Verification items for the finished model (mm, model axes). Face numbers are marked on the shaded views. A direction names the side the tool comes from. Give positions to 0.01 mm unless a question says otherwise; leave off trailing zeros. Write each loop counter-clockwise with the first axis right and the second up, starting at its lowest first coordinate (ties: lowest second). Pieces come first, ordered by that corner, then holes.
from build123d import *

# Parameters (mm, degrees)
BOSS_EXTRUDE1_DEPTH                  = 33.3375
SKETCH3_R                            = 2.0193
CUT_EXTRUDE1_DEPTH                   = 68.328625042
CUT_EXTRUDE3_START                   = -7.9375
SKETCH8_R                            = 6.875
SKETCH8_R_2                          = 6.35
CUT_EXTRUDE3_DEPTH                   = 7.9375
F_10_32_TAPPED_HOLE1_D               = 4.0386
F_10_32_TAPPED_HOLE1_DEPTH           = 12.02944
F_10_32_TAPPED_HOLE1_TIP             = 1.213317848
F_10_32_TAPPED_HOLE1_ON_FACE_2_D     = 4.0386
F_10_32_TAPPED_HOLE1_ON_FACE_2_DEPTH = 12.02944
F_10_32_TAPPED_HOLE1_ON_FACE_2_TIP   = 1.213317848


with BuildPart() as part:
    # Sketch1 → Boss-Extrude1 (new, symmetric)
    with BuildSketch(Plane.XY):
        with BuildLine():
            Line((-0.893039494, 6.816751826), (-5.456960506, 4.181770802))
            ThreePointArc((-5.456960506, 4.181770802), (-5.953924651, 3.4375), (-6.35, 2.634981025))
            Line((-6.35, 2.634981025), (-6.35, -2.634981025))
            ThreePointArc((-6.35, -2.634981025), (-5.953924651, -3.4375), (-5.456960506, -4.181770802))
            Line((-5.456960506, -4.181770802), (-0.893039494, -6.816751826))
            ThreePointArc((-0.893039494, -6.816751826), (0, -6.875), (0.893039494, -6.816751826))
            Line((0.893039494, -6.816751826), (5.456960506, -4.181770802))
            ThreePointArc((5.456960506, -4.181770802), (5.953924651, -3.4375), (6.35, -2.634981025))
            Line((6.35, -2.634981025), (6.35, 2.634981025))
            ThreePointArc((6.35, 2.634981025), (5.953924651, 3.4375), (5.456960506, 4.181770802))
            Line((5.456960506, 4.181770802), (0.893039494, 6.816751826))
            ThreePointArc((0.893039494, 6.816751826), (0, 6.875), (-0.893039494, 6.816751826))
        make_face()
    extrude(amount=BOSS_EXTRUDE1_DEPTH, both=True)

    # Sketch3 → Cut-Extrude1 (cut, through all)
    with BuildSketch(Plane.XY.offset(33.3375)):
        Circle(SKETCH3_R)
    extrude(amount=-CUT_EXTRUDE1_DEPTH, mode=Mode.SUBTRACT)

    # Sketch8 → Cut-Extrude3 (cut)
    with BuildSketch(Plane(origin=(0, 0, -33.3375), x_dir=(-1, 0, 0), z_dir=(0, 0, -1)).offset(CUT_EXTRUDE3_START)):
        Circle(SKETCH8_R)
        with Locations(Location((0, 0, 0), (0, 0, 180))):
            Circle(SKETCH8_R_2, mode=Mode.SUBTRACT)
    extrude(amount=CUT_EXTRUDE3_DEPTH, mode=Mode.SUBTRACT)

    # #10-32 Tapped Hole1
    with Locations(Plane(origin=(0, 0, -33.3375), x_dir=(-1, 0, 0), z_dir=(0, 0, -1))):
        with Locations((0, 0)):
            Hole(F_10_32_TAPPED_HOLE1_D / 2, depth=F_10_32_TAPPED_HOLE1_DEPTH)
            with Locations((0, 0, -(F_10_32_TAPPED_HOLE1_DEPTH + F_10_32_TAPPED_HOLE1_TIP / 2))):  # 118° drill point
                Cone(0, F_10_32_TAPPED_HOLE1_D / 2, F_10_32_TAPPED_HOLE1_TIP, mode=Mode.SUBTRACT)

    # #10-32 Tapped Hole1 on face 2
    with Locations(Plane(origin=(0, 0, 33.3375), x_dir=(-1, 0, 0), z_dir=(0, 0, -1))):
        with Locations((0, 0)):
            Hole(F_10_32_TAPPED_HOLE1_ON_FACE_2_D / 2, depth=F_10_32_TAPPED_HOLE1_ON_FACE_2_DEPTH)
            with Locations((0, 0, -(F_10_32_TAPPED_HOLE1_ON_FACE_2_DEPTH + F_10_32_TAPPED_HOLE1_ON_FACE_2_TIP / 2))):  # 118° drill point
                Cone(0, F_10_32_TAPPED_HOLE1_ON_FACE_2_D / 2, F_10_32_TAPPED_HOLE1_ON_FACE_2_TIP, mode=Mode.SUBTRACT)


solid = part.part
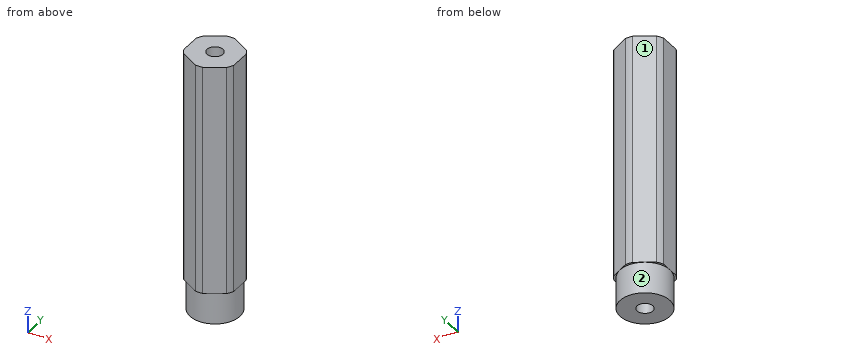
Item 1: Sectioned sample at B-B on z = 8. Record the cut outline in (x, y) (3 decimals), then the cut area to 3 significant figures.
Answer key:
outline: (-6.35, -2.635) arc R6.875 ccw to (-5.457, -4.182) - (-0.893, -6.817) arc R6.875 ccw to (0.893, -6.817) - (5.457, -4.182) arc R6.875 ccw to (6.35, -2.635) - (6.35, 2.635) arc R6.875 ccw to (5.457, 4.182) - (0.893, 6.817) arc R6.875 ccw to (-0.893, 6.817) - (-5.457, 4.182) arc R6.875 ccw to (-6.35, 2.635) - close; hole circle Ø4.039 at (0, 0)
area: 125 mm2
Item 2: Sectioned sample at C-C on y = 3.5. Record the cut outline in (x, z), then the cut area to 3 significant figures.
Answer key:
outline: (-5.92, -25.4) - (-5.3, -25.4) - (-5.3, -33.34) - (5.3, -33.34) - (5.3, -25.4) - (5.92, -25.4) - (5.92, 33.34) - (-5.92, 33.34) - close
area: 779 mm2
Item 3: Scan lines: line 1 along Y through (x, z) = (0, 4) (3 decimals); line 2 along Y through (x, z) = (-1.5, -19); line 3 along X through (y, z) = (1.5, -28). Record each from-to range of solid material in increasing order.
Answer key:
line 1: y = -6.875 to -2.019, 2.019 to 6.875
line 2: y = -6.47 to -1.35, 1.35 to 6.47
line 3: x = -6.17 to -1.35, 1.35 to 6.17
Item 4: Sectioned sample at D-D on x = 4.5. Record the cut outline in (y, z).
Answer key:
outline: (-4.73, -25.4) - (-4.48, -25.4) - (-4.48, -33.34) - (4.48, -33.34) - (4.48, -25.4) - (4.73, -25.4) - (4.73, 33.34) - (-4.73, 33.34) - close
Item 5: Depth check by flat-ended pin: pin 1 (1.5 mm diameter, centred on x = 4.5, z = 11, fed in from +Y); pin 2 (1.5 mm diameter, centred on y = -5.5, z = -26.5, fed in from -X); pin 3 (1 mm diameter, centred on x = -5.5, y = -3.5, fed in from -Z). Enter the tip coordinate at first touch or a pass-through.
Answer key:
pin 1: stops at y = 5.17
pin 2: stops at x = -4.21
pin 3: stops at z = -33.34
Item 6: Set-up check for the marked faces 1 and 2: record each of +Z, -Z, +X, -X, +Y, -Y from which the full face is reachable in a straight line by a thin tool's end or side.
Answer key:
face 1: +Z, -Z, -X, +Y
face 2: -Z
